```python
from build123d import *

# Parameters (mm, degrees)
EXTRUDE_1_DEPTH              = 10
CUT_EXTRUDE_1_DEPTH          = 34.383433003
FILLET_1_SIZE                = 4
FILLET_1_SIZE_2              = 6
CUT_EXTRUDE_2_DEPTH          = 34.383433056
CUT_EXTRUDE_2_DEPTH_BACK     = 34.383433056
SKETCH_3_W                   = 58.405721138
SKETCH_3_H                   = 2.2
SKETCH_4_W                   = 2.75
SKETCH_4_H                   = 7.7
EXTRUDE_2_DEPTH              = 7.35
SKETCH_5_R                   = 0.75
CUT_EXTRUDE_3_DEPTH          = 54.030431013
FILLET_2_R                   = 3.85
CORTAR_EXTRUIR1_DEPTH        = 33.791669707
SALIENTE_EXTRUIR1_DEPTH      = 7.7
CROQUIS2_R                   = 20
CORTAR_EXTRUIR3_DEPTH        = 35.438086687
SALIENTE_EXTRUIR4_DEPTH      = 7
SALIENTE_EXTRUIR4_DEPTH_BACK = 7
CORTAR_EXTRUIR4_DEPTH        = 37.368830262
REDONDEO3_R                  = 2
REDONDEO4_R                  = 10


# Some blends are built 0.0001 mm under size
with BuildPart() as part:
    # 草图1 → 凸台-拉伸1 (new body)
    with BuildSketch(Plane(origin=(0, 0, 0), x_dir=(1, 0, 0), z_dir=(0, 1, 0))):
        Polygon((27.5, 3.85), (-27.5, 3.85), (-29.64, 3.85), (-30.905721138, 2.584278862), (-29.70363961, 1.382197334), (-28.935836944, 2.15), (-27.5, 2.15), (-27.5, -2.15), (-29.64, -2.15), (-30.905721138, -3.415721138), (-29.70363961, -4.617802666), (-28.935836944, -3.85), (-27.5, -3.85), (27.5, -3.85), align=None)
    extrude(amount=EXTRUDE_1_DEPTH)

    # 草图2 → 切除-拉伸1 (cut, through all)
    with BuildSketch(Plane.XY.offset(3.85)):
        with BuildLine():
            Line((-18.935836944, 0), (21.5, 0))
            ThreePointArc((21.5, 0), (1.282081528, 3.70613757), (-18.935836944, 0))
        make_face()
    extrude(amount=-CUT_EXTRUDE_1_DEPTH, mode=Mode.SUBTRACT)

    # 圆角1
    # an asymmetric fillet: 6, 4 mm, written as the material it takes off along each edge
    with BuildSketch(Plane(origin=(27.5, 0, 18.85), x_dir=(-1, 0, 0), z_dir=(0, 0, -1))) as fillet_1_piece_1:
        with BuildLine():
            Bezier((FILLET_1_SIZE, 0), (0, 0), (0, FILLET_1_SIZE_2), weights=[1, 0.707106781, 1])
            Line((0, FILLET_1_SIZE_2), (0, 0))
            Line((0, 0), (FILLET_1_SIZE, 0))
        make_face()
    extrude(amount=37.7, mode=Mode.SUBTRACT)

    # 草图3 → 切除-拉伸2 (cut, two sides: drawn at the far end of the back side and taken through both)
    with BuildSketch(Plane.XY.offset(3.85).offset(-CUT_EXTRUDE_2_DEPTH_BACK)):
        with Locations((-1.702860569, 8.9)):
            Rectangle(SKETCH_3_W, SKETCH_3_H)
    extrude(amount=CUT_EXTRUDE_2_DEPTH + CUT_EXTRUDE_2_DEPTH_BACK, mode=Mode.SUBTRACT)

    # 草图4 → 凸台-拉伸2 (add)
    with BuildSketch(Plane.XZ):
        with Locations((-26.125, 0)):
            Rectangle(SKETCH_4_W, SKETCH_4_H)
    extrude(amount=EXTRUDE_2_DEPTH)

    # 草图5 → 切除-拉伸3 (cut, through all)
    with BuildSketch(Plane(origin=(-24.75, 0, 0), x_dir=(0, 0, -1), z_dir=(1, 0, 0))):
        with Locations((0, -3.5)):
            Circle(SKETCH_5_R)
    extrude(amount=-CUT_EXTRUDE_3_DEPTH, mode=Mode.SUBTRACT)

    # 圆角2
    fillet_2_edges = [part.edges().sort_by_distance(p)[0] for p in [
        (-26.125, -7.35, -3.85),
        (-26.125, -7.35, 3.85),
    ]]
    fillet(fillet_2_edges, radius=FILLET_2_R - 0.0001)  # a hair under: the kernel refuses the full size

    # Croquis1 → Cortar-Extruir1 (cut, through all)
    with BuildSketch(Plane.XY.offset(3.85)):
        with BuildLine():
            Line((27.5, 7.8), (16.217886534, 7.8))
            Line((16.217886534, 7.8), (23.5, 2.765439303))
            Line((23.5, 2.765439303), (23.5, 0))
            add(Edge.make_bspline(
                [(27.5, 6), (27.5, 5.69042848), (27.487576866, 5.380787378), (27.462721246, 5.071641684), (27.425314756, 4.763619555), (27.375158046, 4.457411018), (27.311958659, 4.153772273), (27.15893131, 3.554601129), (27.069254161, 3.259173226), (26.965810638, 2.96797603), (26.848060748, 2.682057947), (26.71538748, 2.402788295), (26.567124674, 2.131846167), (26.305522028, 1.71806679), (26.202980384, 1.568477856), (26.094611251, 1.422961788), (25.980267973, 1.282053299), (25.859832084, 1.146386576), (25.733223411, 1.016687557), (25.50418613, 0.80470891), (25.40471615, 0.719219867), (25.301997411, 0.637611459), (25.196057574, 0.56023543), (25.086963249, 0.487470604), (24.97482846, 0.419710585), (24.681074838, 0.260429148), (24.49523869, 0.176468902), (24.303178892, 0.107130148), (24.106026723, 0.053886894), (23.905206432, 0.017937167), (23.702478464, 0), (23.5, 0)],
                knots=[0, 0, 0, 0, 0, 0, 0, 0, 0.272858712, 0.272858712, 0.272858712, 0.272858712, 0.272858712, 0.272858712, 0.544533939, 0.544533939, 0.544533939, 0.544533939, 0.544533939, 0.544533939, 0.704314184, 0.704314184, 0.704314184, 0.704314184, 0.704314184, 0.704314184, 0.820075996, 0.820075996, 0.820075996, 0.820075996, 0.820075996, 0.820075996, 1, 1, 1, 1, 1, 1, 1, 1], degree=7))
            Line((27.5, 6), (27.5, 7.8))
        make_face()
    extrude(amount=-CORTAR_EXTRUIR1_DEPTH, mode=Mode.SUBTRACT)

    # Croquis1<3> → Saliente-Extruir1 (add)
    with BuildSketch(Plane.XY.offset(3.85)):
        Polygon((-24.75, 13.096878085), (-24.75, 7.8), (16.217886534, 7.8), (8.556350692, 13.096878085), align=None)
        with BuildLine():
            ThreePointArc((21.5, 0), (1.282081528, 3.70613757), (-18.935836944, 0))
            Line((-18.935836944, 0), (21.5, 0))
        make_face()
        with BuildLine():
            Line((-24.75, 7.8), (-24.75, 0))
            Line((-24.75, 0), (-18.935836944, 0))
            ThreePointArc((-18.935836944, 0), (1.282081528, 3.70613757), (21.5, 0))
            Line((21.5, 0), (23.5, 0))
            Line((23.5, 0), (23.5, 2.765439303))
            Line((23.5, 2.765439303), (16.217886534, 7.8))
            Line((16.217886534, 7.8), (-24.75, 7.8))
        make_face()
    extrude(amount=-SALIENTE_EXTRUIR1_DEPTH)

    # Croquis2 → Cortar-Extruir3 (cut, through all)
    with BuildSketch(Plane.XY.offset(3.85)):
        with Locations((1.282081528, -12.8)):
            Circle(CROQUIS2_R)
    extrude(amount=-CORTAR_EXTRUIR3_DEPTH, mode=Mode.SUBTRACT)

    # Croquis3 → Saliente-Extruir4 (add, two sides: drawn at the far end of the back side and taken through both)
    with BuildSketch(Plane.XY.offset(-SALIENTE_EXTRUIR4_DEPTH_BACK)):
        with BuildLine():
            ThreePointArc((16.649579698, 0), (1.282081528, 7.2), (-14.085416642, 0))
            Line((-14.085416642, 0), (-24.75, 0))
            Line((-24.75, 0), (-24.75, 7.8))
            Line((-24.75, 7.8), (-24.75, 13.096878085))
            Line((-24.75, 13.096878085), (8.556350692, 13.096878085))
            Line((8.556350692, 13.096878085), (23.5, 2.765439303))
            Line((23.5, 2.765439303), (23.5, 0))
            Line((23.5, 0), (16.649579698, 0))
        make_face()
        with BuildLine():
            Line((16.649579698, 0), (-14.085416642, 0))
            ThreePointArc((-14.085416642, 0), (1.282081528, 7.2), (16.649579698, 0))
        make_face()
    extrude(amount=SALIENTE_EXTRUIR4_DEPTH + SALIENTE_EXTRUIR4_DEPTH_BACK)

    # Croquis4 → Cortar-Revolución2 (revolve, cut)
    with BuildSketch(Plane.XY):
        with BuildLine():
            ThreePointArc((14.588399238, 2.131239365), (1.282081528, 7.2), (-12.024236182, 2.131239365))
            ThreePointArc((-12.024236182, 2.131239365), (1.282081528, 3.70613757), (14.588399238, 2.131239365))
        make_face()
        with BuildLine():
            ThreePointArc((-12.024236182, 2.131239365), (-13.094374036, 1.103867282), (-14.085416642, 0))
            Line((-14.085416642, 0), (16.649579698, 0))
            ThreePointArc((16.649579698, 0), (15.658537092, 1.103867282), (14.588399238, 2.131239365))
            ThreePointArc((14.588399238, 2.131239365), (1.282081528, 3.70613757), (-12.024236182, 2.131239365))
        make_face()
    revolve(axis=Axis((1.282081528, -12.8, 0), (-1, 0, 0)), mode=Mode.SUBTRACT)

    # Croquis5 → Cortar-Extruir4 (cut, through all)
    with BuildSketch(Plane.XY.offset(7)):
        Polygon((-22.59131667, 0), (-21.246710257, -0.018288841), (-21.903174863, 1.155318891), align=None)
        Polygon((-24.39131667, 0), (-23.046710257, -0.018288841), (-23.703174863, 1.155318891), align=None)
        Polygon((-20.79131667, 0), (-19.446710257, -0.018288841), (-20.103174863, 1.155318891), align=None)
        Polygon((-18.99131667, 0), (-17.646710257, -0.018288841), (-18.303174863, 1.155318891), align=None)
        Polygon((-17.19131667, 0), (-15.846710257, -0.018288841), (-16.503174863, 1.155318891), align=None)
        Polygon((-15.39131667, 0), (-14.046710257, -0.018288841), (-14.703174863, 1.155318891), align=None)
        Polygon((17.00868333, 0), (18.353289743, -0.018288841), (17.696825137, 1.155318891), align=None)
        Polygon((18.80868333, 0), (20.153289743, -0.018288841), (19.496825137, 1.155318891), align=None)
        Polygon((20.60868333, 0), (21.953289743, -0.018288841), (21.296825137, 1.155318891), align=None)
    extrude(amount=-CORTAR_EXTRUIR4_DEPTH, mode=Mode.SUBTRACT)

    # Redondeo3
    redondeo3_edges = [part.edges().sort_by_distance(p)[0] for p in [
        (23.5, 2.765439303, 0),
        (-24.75, 13.096878085, 0),
    ]]
    fillet(redondeo3_edges, radius=REDONDEO3_R)

    # Redondeo4
    redondeo4_edges = [part.edges().sort_by_distance(p)[0] for p in [
        (8.556350692, 13.096878085, 0),
    ]]
    fillet(redondeo4_edges, radius=REDONDEO4_R)


solid = part.part
```
Design review of the part built by this model. Coordinates are the model's own, in mm. A direction names the side the tool comes from. Coordinates: 2 decimals unless noted, no trailing zeros. Order: outer loops, then holes, each group sorted by start corner. A loop starts at its lowest first (then second) coordinate and runs counter-clockwise, first axis right, second up. Notation, with made-up numbers: M 11,-5 L 33,-5 A27 ccw 33,24 Z; hole C 73.5,-39 d7. An arc over 180 degrees is marked long. Answer as a JSON object with one key per item and string values. Group by question number.
1) For pin 1 (2 mm diameter, centred on x = -29, z = 4, fed in from -Y); pin 2 (1.1 mm diameter, centred on x = -28.5, y = 4, fed in from -Z); pin 3 (3.5 mm diameter, centred on y = 7.5, z = 1, fed in from -X), all flat-tipped, find the tip position at first contact; note any pin that passes through.
2) Tool access review of faces 4 (the flat face through (-9, 13.097, 0)), 5 (the flat face through (-29, 4, 2.15)), 6 (the cylindrical face through (-26.106, -6.252, 2.692)), 7 (the flat face through (-29, 0, -3)), 8 (the flat face through (-28, 4, -2.15)): name each direction out of +Z, -Z, +X, -X, +Y, -Y from which nothing blocks a thin tool from reaching the whole face with its end or side.
3) Add section B-B, the plane x = 0. Write out the cut boundary in (y, z).
4) Add section A-A, the plane y = 4.5. Write out the cut boundary in (x, z), then the cut area to 3 significant figures.
5) Add section C-C, the plane y = 10.5. Write out the cut boundary in (x, z).
6) Mouldability with a two-part tool opening along X and no side actions: class faces 1 (the flat face through (-27, 7.8, 0)), 2 (the flat face through (-17.976, 0.57, 0.098)), 3 (the flat face through (23.5, 1, 0)) as pulls with the +X half, pulls with the -X half, needs draft (parallel to the pull), parting line crosses it, or undercut.
7) Add section D-D, the plane y = -5. Write out the cut boundary in (x, z), then the cut area to 3 significant figures.
8) Wall thickness on L1, parallel to Y at x = -26.45, z = 0; L2, parallel to X at y = 4.5, z = -2; L3, parallel to Y at x = -27, z = -0.5: over which ranges is each line inside the solid? List them lowest first.
Computed values:
{
 "1": {"pin 1": "stops at y = 0", "pin 2": "stops at z = -3.85", "pin 3": "stops at x = -30.24"},
 "2": {"face 4": "+Z, -Z, +X, -X, +Y", "face 5": "-X, +Y, -Y", "face 6": "+Z, +X, -X, -Y", "face 7": "+Z, -Z, -X, -Y", "face 8": "+Y, -Y"},
 "3": {"outline": "M 5.89,-7 L 13.1,-7 L 13.1,7 L 5.89,7 A19.96 cw Z"},
 "4": {"outline": "M -30.91,-2.58 L -29.64,-3.85 L -24.75,-3.85 L -24.75,-7 L -5.91,-7 A10.04 cw -5.91,7 L -24.75,7 L -24.75,3.85 L -28.94,3.85 L -29.7,4.62 L -30.91,3.42 L -29.64,2.15 L -27.5,2.15 L -27.5,-2.15 L -28.94,-2.15 L -29.7,-1.38 Z; M 8.47,-7 L 20.99,-7 L 20.99,7 L 8.47,7 A10.04 cw Z", "area": "416 mm^2"},
 "5": {"outline": "M -24.75,-7 L 12.31,-7 L 12.31,7 L -24.75,7 Z"},
 "6": {"face 1": "needs draft", "face 2": "undercut", "face 3": "pulls with the +X half"},
 "7": {"outline": "M -27.5,-3.55 L -24.75,-3.55 L -24.75,3.55 L -27.5,3.55 Z", "area": "19.5 mm^2"},
 "8": {"L1": "y = -7.35 to -4.25, -2.75 to 7.8", "L2": "x = -30.32 to -29.09, -27.5 to -8.55, 11.12 to 20.99", "L3": "y = -7.32 to -4.06, -2.94 to 7.8"}
}
